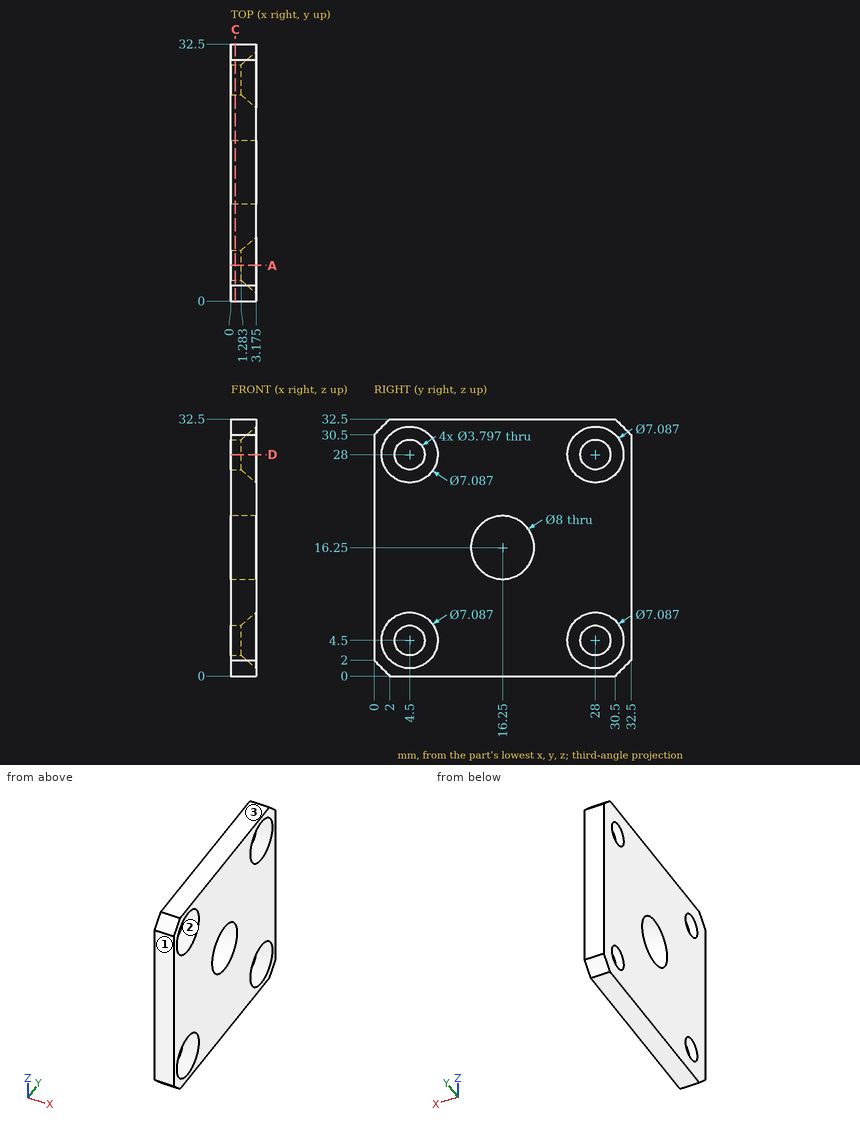
Could you check a few things on this drawing? It's one solid part, dimensions in mm from its lowest x, y, z. Coordinates: 2 decimals unless noted, no trailing zeros. Write each loop counter-clockwise with the first axis right and the second up, starting at its lowest first coordinate (ties: lowest second). Pieces come first, ordered by that corner, then holes. Notation, with made-up numbers: (70, -28) - (75, -28) arc R8 cw to (75, -20) - close; hole circle Ø3 at (37.25, 12.5). An arc over 180 degrees is marked (long way). Put each result on its own line as item: value. Start each with the question number.
Q1. I'm going to push a flat-ended pin straight in: P1, Ø6, axis at y = 28, z = 4.5, coming from the +X side. Where does the tip first touch, or does it pass through?
Q2. I want a section at A-A on y = 4.5. Write out the boundary of the cut face in (x, z) (1 decimal).
Q3. Please list where these lines run through material, in increasing order: L1, parallel to Z at x = 0.3, y = 28; L2, parallel to Y at x = 1.7, z = 16.25.
Q4. Thinking about a two-plate mould opening in Z: for the marked faces 1, 2 and 3, which applies, pulls with the +Z half, pulls with the -Z half, needs draft (parallel to the pull), parting line crosses it, or undercut?
Q5. I want a section at C-C on x = 0.55. Write out the boundary of the cut face in (y, z), plus the area to 3 significant figures.
Checks:
1. P1: x = 2.55
2. outline: (0, 0) - (3.2, 0) - (3.2, 1) - (1.3, 2.6) - (0, 2.6) - close; (0, 6.4) - (1.3, 6.4) - (3.2, 8) - (3.2, 24.5) - (1.3, 26.1) - (0, 26.1) - close; (0, 29.9) - (1.3, 29.9) - (3.2, 31.5) - (3.2, 32.5) - (0, 32.5) - close
3. L1: 0 to 2.6, 6.4 to 26.1, 29.9 to 32.5
3. L2: 0 to 12.25, 20.25 to 32.5
4. face 1: needs draft
4. face 2: undercut
4. face 3: pulls with the +Z half
5. outline: (0, 2) - (2, 0) - (30.5, 0) - (32.5, 2) - (32.5, 30.5) - (30.5, 32.5) - (2, 32.5) - (0, 30.5) - close; hole circle Ø3.8 at (4.5, 4.5); hole circle Ø3.8 at (4.5, 28); hole circle Ø8 at (16.25, 16.25); hole circle Ø3.8 at (28, 4.5); hole circle Ø3.8 at (28, 28)
5. area: 953 mm²
